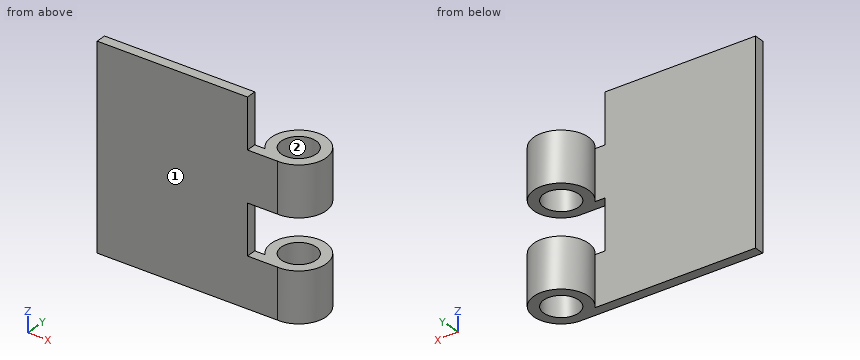
```python
from build123d import *

# Parameters (mm, degrees)
BOSS_EXTRUDE1_DEPTH = 1
SKETCH2_R           = 2.75
SKETCH2_R_2         = 1.75
BOSS_EXTRUDE2_DEPTH = 5
SKETCH3_R           = 2.75
SKETCH3_R_2         = 1.75
BOSS_EXTRUDE3_DEPTH = 5


with BuildPart() as part:
    # Sketch1 → Boss-Extrude1 (new body)
    with BuildSketch(Plane(origin=(0, 0, 0), x_dir=(1, 0, 0), z_dir=(0, 1, 0))):
        Polygon((0, 10), (0, -10), (15, -10), (15, -5), (18, -5), (18, 0), (15, 0), (15, 5), (18, 5), (18, 10), align=None)
    extrude(amount=-BOSS_EXTRUDE1_DEPTH)

    # Sketch2 → Boss-Extrude2 (add)
    with BuildSketch(Plane(origin=(0, 0, -10), x_dir=(-1, 0, 0), z_dir=(0, 0, -1))):
        with Locations((-18.130154704, 1.75)):
            Circle(SKETCH2_R)
        with Locations((-18.130154704, 1.75)):
            Circle(SKETCH2_R_2, mode=Mode.SUBTRACT)
    extrude(amount=-BOSS_EXTRUDE2_DEPTH)

    # Sketch3 → Boss-Extrude3 (add)
    with BuildSketch(Plane(origin=(0, 0, 0), x_dir=(-1, 0, 0), z_dir=(0, 0, -1))):
        with Locations((-18.130154704, 1.75)):
            Circle(SKETCH3_R)
        with Locations((-18.130154704, 1.75)):
            Circle(SKETCH3_R_2, mode=Mode.SUBTRACT)
    extrude(amount=-BOSS_EXTRUDE3_DEPTH)


solid = part.part
```
Verification items for the finished model (mm, model axes). Face numbers are marked on the shaded views. Coordinates: 2 decimals unless noted, no trailing zeros. Order: outer loops, then holes, each group sorted by start corner. A loop starts at its lowest first (then second) coordinate and runs counter-clockwise, first axis right, second up. Notation, with made-up numbers: (82, 19) - (89, 19) arc R36 cw to (89, 56) - close; hole circle Ø9 at (38, 30). An arc over 180 degrees is marked (long way). Return JSON: item names as keys, results as strings.
(1) Section check D-D, the plane y = 2.8. Record the cut outline in (x, z), and give its area (3 significant figures).
Filled sheet:
{"outline": "(15.59, -10) - (16.73, -10) - (16.73, -5) - (15.59, -5) - close; (15.59, 0) - (16.73, 0) - (16.73, 5) - (15.59, 5) - close; (19.53, -10) - (20.67, -10) - (20.67, -5) - (19.53, -5) - close; (19.53, 0) - (20.67, 0) - (20.67, 5) - (19.53, 5) - close", "area": "22.8 mm^2"}
(2) Section check C-C, the plane x = 9.75. Record the cut outline in (y, z).
Filled sheet:
{"outline": "(-1, -10) - (0, -10) - (0, 10) - (-1, 10) - close"}
(3) Mould release check, pull along Y, two halves, no side actions. Record for the marked faces 1 and 2: pulls with the +Y half, pulls with the -Y half, needs draft (parallel to the pull), parting line crosses it, or undercut.
Filled sheet:
{"face 1": "pulls with the -Y half", "face 2": "undercut"}
(4) Thickness scan on line 1 along Y through (x, z) = (13, -8.75); line 2 along Y through (x, z) = (18.5, -8.5); line 3 along X through (y, z) = (2.2, 0.75). Record the ranges inside material, lowest first.
Filled sheet:
{"line 1": "y = -1 to 0", "line 2": "y = -0.98 to 0.04, 3.46 to 4.48", "line 3": "x = 15.42 to 16.44, 19.82 to 20.84"}
(5) Go/stop test with flat-tipped pins: pin 1 (1.5 mm diameter, centred on y = 1.5, z = -4.5, fed in from -X); pin 2 (0.8 mm diameter, centred on y = -0.5, z = 7, fed in from +X). Record where each tip stops, or that it passes through.
Filled sheet:
{"pin 1": "stops at x = 15.38", "pin 2": "stops at x = 15"}
(6) Section check A-A, the plane y = 1.75. Record the cut outline in (x, z), and give its area (3 significant figures).
Filled sheet:
{"outline": "(15.38, -10) - (16.38, -10) - (16.38, -5) - (15.38, -5) - close; (15.38, 0) - (16.38, 0) - (16.38, 5) - (15.38, 5) - close; (19.88, -10) - (20.88, -10) - (20.88, -5) - (19.88, -5) - close; (19.88, 0) - (20.88, 0) - (20.88, 5) - (19.88, 5) - close", "area": "20.0 mm^2"}
